```python
from build123d import *

# Parameters (mm, degrees)
BOSS_EXTRUDE1_START             = -711.2
SKETCH5_W                       = 19.05
SKETCH5_H                       = 19.05
SKETCH5_R                       = 5
BOSS_EXTRUDE1_DEPTH             = 25.4
F_5_0MM_DOWEL_HOLE2_D           = 5
F_5_0MM_DOWEL_HOLE2_DEPTH       = 25.4
F_5_0MM_DOWEL_HOLE2_CSINK_D     = 5.05
F_5_0MM_DOWEL_HOLE2_CSINK_ANGLE = 90
F_5_0MM_DOWEL_HOLE2_TIP         = 1.502151548
F_3_0MM_DOWEL_HOLE2_D           = 3
F_3_0MM_DOWEL_HOLE2_DEPTH       = 12.7
F_3_0MM_DOWEL_HOLE2_CSINK_D     = 3.05
F_3_0MM_DOWEL_HOLE2_CSINK_ANGLE = 90
F_3_0MM_DOWEL_HOLE2_TIP         = 0.901290929


with BuildPart() as part:
    # Sketch5 → Boss-Extrude1 (new body)
    with BuildSketch(Plane.XY.offset(BOSS_EXTRUDE1_START)):
        with Locations((63.5, 83.82)):
            Rectangle(SKETCH5_W, SKETCH5_H)
        with Locations((63.5, 83.82)):
            Circle(SKETCH5_R, mode=Mode.SUBTRACT)
    extrude(amount=BOSS_EXTRUDE1_DEPTH)

    # Ø5.0mm Dowel Hole2
    with Locations(Plane(origin=(0, 93.345, 0), x_dir=(1, 0, 0), z_dir=(0, 1, 0))):
        with Locations((57.15, 692.15), (69.85, 692.15)):
            CounterSinkHole(F_5_0MM_DOWEL_HOLE2_D / 2, F_5_0MM_DOWEL_HOLE2_CSINK_D / 2, depth=F_5_0MM_DOWEL_HOLE2_DEPTH, counter_sink_angle=F_5_0MM_DOWEL_HOLE2_CSINK_ANGLE)
            with Locations((0, 0, -(F_5_0MM_DOWEL_HOLE2_DEPTH + F_5_0MM_DOWEL_HOLE2_TIP / 2))):  # 118° drill point
                Cone(0, F_5_0MM_DOWEL_HOLE2_D / 2, F_5_0MM_DOWEL_HOLE2_TIP, mode=Mode.SUBTRACT)

    # Ø3.0mm Dowel Hole2
    with Locations(Plane(origin=(0, 0, -711.2), x_dir=(-1, 0, 0), z_dir=(0, 0, -1))):
        with Locations((-58.42, 78.74), (-68.58, 78.74), (-58.42, 88.9), (-68.58, 88.9)):
            CounterSinkHole(F_3_0MM_DOWEL_HOLE2_D / 2, F_3_0MM_DOWEL_HOLE2_CSINK_D / 2, depth=F_3_0MM_DOWEL_HOLE2_DEPTH, counter_sink_angle=F_3_0MM_DOWEL_HOLE2_CSINK_ANGLE)
            with Locations((0, 0, -(F_3_0MM_DOWEL_HOLE2_DEPTH + F_3_0MM_DOWEL_HOLE2_TIP / 2))):  # 118° drill point
                Cone(0, F_3_0MM_DOWEL_HOLE2_D / 2, F_3_0MM_DOWEL_HOLE2_TIP, mode=Mode.SUBTRACT)


solid = part.part
```
Geometry check sheet. Reference: the model listing, model coordinates, mm. A direction names the side the tool comes from. Coordinates: 2 decimals unless noted, no trailing zeros. Order: outer loops, then holes, each group sorted by start corner. A loop starts at its lowest first (then second) coordinate and runs counter-clockwise, first axis right, second up. Notation, with made-up numbers: M 12,-25 L 23,-25 A28 cw 23,-3 Z; hole C 28,-16 d3. An arc over 180 degrees is marked long. Answer as a JSON object with one key per item and string values.
Q1. Tool access check on faces 1 (the cylindrical face through (59.806, 78.165, -704.749)), 2 (the cylindrical face through (72.348, 83.674, -692.26)). Record the directions out of +Z, -Z, +X, -X, +Y, -Y that give a thin tool (end or side, any length) a straight path to the whole face; none if there is none.
Results are:
{"face 1": "-Z", "face 2": "+Y, -Y"}
Q2. Cross-section at A-A on z = -700. Record the cut outline in (x, y) (3 decimals), and give its area (3 significant figures).
Results are:
{"outline": "M 53.975,74.295 L 73.025,74.295 L 73.025,93.345 L 53.975,93.345 Z; hole C 58.42,78.74 d3; hole C 58.42,88.9 d3; hole C 63.5,83.82 d10; hole C 68.58,78.74 d3; hole C 68.58,88.9 d3", "area": "256 mm²"}
Q3. Depth check by flat-ended pin: pin 1 Ø2.5 at (x, y) = (68.58, 88.9) entering from -Z; pin 2 Ø1.8 at (x, y) = (58.42, 78.74) entering from -Z. Enter the tip coordinate at first touch or a pass-through.
Results are:
{"pin 1": "stops at z = -698.35", "pin 2": "stops at z = -698.14"}
Q4. Scan lines: line 1 (X direction, y = 78.74, z = -706.75) (3 decimals); line 2 (Y direction, x = 68.58, z = -704.75) (3 decimals); line 3 (Y direction, x = 63.5, z = -702.25) (3 decimals). Record each from-to range of solid material in increasing order.
Results are:
{"line 1": "x = 53.975 to 56.92, 59.92 to 67.08, 70.08 to 73.025", "line 2": "y = 74.295 to 77.24, 80.24 to 87.4, 90.4 to 93.345", "line 3": "y = 74.295 to 78.82, 88.82 to 93.345"}
Q5. Release check for a two-part mould opening along X. For faces 3 (the flat face through (63, 74.295, -699)), 4 (the conical face through (58.454, 78.998, -697.755)), 5 (the flat face through (53.975, 84, -699)) record: released by +X, released by -X, zero draft, split by the parting line, or undercut.
Results are:
{"face 3": "zero draft", "face 4": "undercut", "face 5": "released by -X"}
Q6. Cross-section at B-B on x = 65.5. Record the cut outline in (y, z) (3 decimals), and give its area (3 significant figures).
Results are:
{"outline": "M 74.295,-711.2 L 79.237,-711.2 L 79.237,-685.8 L 74.295,-685.8 Z; M 88.403,-711.2 L 93.345,-711.2 L 93.345,-685.8 L 88.403,-685.8 Z", "area": "251 mm²"}
Q7. Cross-section at C-C on y = 91.5. Record the cut outline in (x, z) (3 decimals), and give its area (3 significant figures).
Results are:
{"outline": "M 53.975,-711.2 L 73.025,-711.2 L 73.025,-685.8 L 53.975,-685.8 Z; hole C 57.15,-692.15 d5; hole C 69.85,-692.15 d5", "area": "445 mm²"}
Q8. Cross-section at D-D on z = -696.25. Record the cut outline in (x, y) (3 decimals).
Results are:
{"outline": "M 53.975,74.295 L 73.025,74.295 L 73.025,93.345 L 53.975,93.345 Z; hole C 63.5,83.82 d10"}
